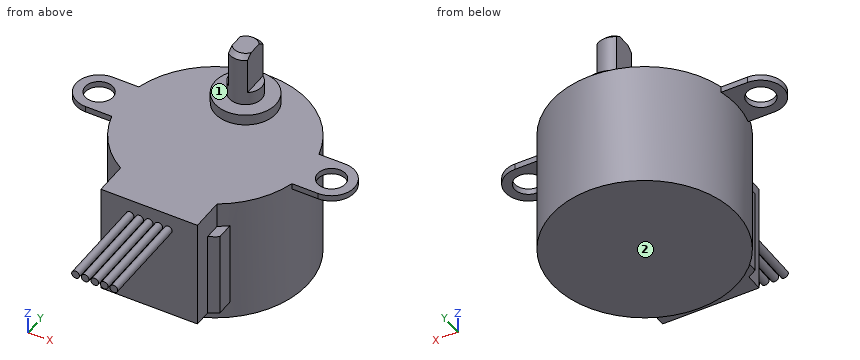
```python
from build123d import *

# Parameters (mm, degrees)
SKETCH1_R           = 14
BOSS_EXTRUDE1_DEPTH = 19.2
BOSS_EXTRUDE2_DEPTH = 16.64
BOSS_EXTRUDE3_DEPTH = 12.87
SKETCH4_R           = 0.585
BOSS_EXTRUDE4_DEPTH = 14
SKETCH5_R           = 4.6
BOSS_EXTRUDE5_DEPTH = 1.63
SKETCH6_R           = 2.445
BOSS_EXTRUDE6_DEPTH = 8.1
CUT_EXTRUDE1_DEPTH  = 6.08
CHAMFER1_SIZE       = 0.68
SKETCH8_R           = 2.1
BOSS_EXTRUDE7_DEPTH = 0.9


with BuildPart() as part:
    # Sketch1 → Boss-Extrude1 (new body)
    with BuildSketch(Plane.XY):
        Circle(SKETCH1_R)
    extrude(amount=-BOSS_EXTRUDE1_DEPTH)

    # Sketch2 → Boss-Extrude2 (add)
    with BuildSketch(Plane.XY):
        with BuildLine():
            Line((-7.265, -11.967446469), (-7.265, -17))
            Line((-7.265, -17), (7.265, -17))
            Line((7.265, -17), (7.265, -11.967446469))
            ThreePointArc((7.265, -11.967446469), (0, -14), (-7.265, -11.967446469))
        make_face()
    extrude(amount=-BOSS_EXTRUDE2_DEPTH)

    # Sketch3 → Boss-Extrude3 (add)
    with BuildSketch(Plane(origin=(0, 0, -16.64), x_dir=(-1, 0, 0), z_dir=(0, 0, -1))):
        with BuildLine():
            Line((7.265, -14.390072098), (7.265, -11.967446469))
            ThreePointArc((7.265, -11.967446469), (7.969331726, -11.510419273), (8.645, -11.011992327))
            Line((8.645, -11.011992327), (8.645, -13.605821364))
            ThreePointArc((8.645, -13.605821364), (7.964658643, -14.014942479), (7.265, -14.390072098))
        make_face()
        with BuildLine():
            Line((-7.265, -11.967446469), (-7.265, -14.390072098))
            ThreePointArc((-7.265, -14.390072098), (-7.964658643, -14.014942479), (-8.645, -13.605821364))
            Line((-8.645, -13.605821364), (-8.645, -11.011992327))
            ThreePointArc((-8.645, -11.011992327), (-7.969331726, -11.510419273), (-7.265, -11.967446469))
        make_face()
    extrude(amount=-BOSS_EXTRUDE3_DEPTH)

    # Sketch4 → Boss-Extrude4 (add)
    with BuildSketch(Plane.XZ.offset(17)):
        with Locations((-2.88, -2.555)):
            Circle(SKETCH4_R)
        with Locations((-1.44, -2.555)):
            Circle(SKETCH4_R)
        with Locations((0, -2.555)):
            Circle(SKETCH4_R)
        with Locations((1.44, -2.555)):
            Circle(SKETCH4_R)
        with Locations((2.88, -2.555)):
            Circle(SKETCH4_R)
    extrude(amount=BOSS_EXTRUDE4_DEPTH)

    # Sketch5 → Boss-Extrude5 (add)
    with BuildSketch(Plane.XY):
        with Locations((0, 7.77)):
            Circle(SKETCH5_R)
    extrude(amount=BOSS_EXTRUDE5_DEPTH)

    # Sketch6 → Boss-Extrude6 (add)
    with BuildSketch(Plane.XY.offset(1.63)):
        with Locations((0, 7.77)):
            Circle(SKETCH6_R)
    extrude(amount=BOSS_EXTRUDE6_DEPTH)

    # Sketch7 → Cut-Extrude1 (cut)
    with BuildSketch(Plane.XY.offset(9.73)):
        with BuildLine():
            Line((1.44, 9.745961791), (1.44, 5.794038209))
            ThreePointArc((1.44, 5.794038209), (2.445, 7.77), (1.44, 9.745961791))
        make_face()
        with BuildLine():
            Line((-1.44, 9.745961791), (-1.44, 5.794038209))
            ThreePointArc((-1.44, 5.794038209), (-2.445, 7.77), (-1.44, 9.745961791))
        make_face()
    extrude(amount=-CUT_EXTRUDE1_DEPTH, mode=Mode.SUBTRACT)

    # Chamfer1
    chamfer1_edges = [part.edges().sort_by_distance(p)[0] for p in [
        (0, 10.215, 9.73),
        (0, 5.325, 9.73),
    ]]
    chamfer(chamfer1_edges, length=CHAMFER1_SIZE)

    # Sketch8 → Boss-Extrude7 (add)
    with BuildSketch(Plane.XY):
        with BuildLine():
            Line((-13.561872105, 3.475), (-17.5, 3.475))
            ThreePointArc((-17.5, 3.475), (-20.975, 0), (-17.5, -3.475))
            Line((-17.5, -3.475), (-13.561872105, -3.475))
            ThreePointArc((-13.561872105, -3.475), (-14, 0), (-13.561872105, 3.475))
        make_face()
        with Locations((-17.5, 0)):
            Circle(SKETCH8_R, mode=Mode.SUBTRACT)
        with BuildLine():
            Line((17.5, -3.475), (13.561872105, -3.475))
            ThreePointArc((13.561872105, -3.475), (14, 0), (13.561872105, 3.475))
            Line((13.561872105, 3.475), (17.5, 3.475))
            ThreePointArc((17.5, 3.475), (20.975, 0), (17.5, -3.475))
        make_face()
        with Locations((17.5, 0)):
            Circle(SKETCH8_R, mode=Mode.SUBTRACT)
    extrude(amount=-BOSS_EXTRUDE7_DEPTH)


solid = part.part
```
Work out the finished part from the listing and answer in its coordinate system (mm). Face numbers are marked on the shaded views. A direction names the side the tool comes from. Give positions to 0.01 mm unless a question says otherwise; leave off trailing zeros. Loops run counter-clockwise (first coordinate to the right, second up) from the corner with the lowest first, then second, coordinate; pieces in that order, holes last. Notation, with made-up numbers: M 89.25,1 L 102.25,1 A25 cw 102.25,25 Z; hole C -12,-31 d9. An arc over 180 degrees is marked long. One line per item, written item: value. Start each with the question number.
1. Each of these flat-tipped pins is pushed along its axis until it touches: P1, Ø5, axis at y = 6, z = -6.5, coming from the -X side; P2, Ø1, axis at x = 16, z = -0.5, coming from the +Y side (3 decimals); P3, Ø2.5, axis at y = -15.5, z = -7.5, coming from the +X side. Where does it stop, or does it pass through?
2. Find the intervals of material crossed by probe 1 along Z at (x, y) = (-8, -2); probe 2 along Y at (x, z) = (-17.5, -0.35) (3 decimals); probe 3 along X at (y, z) = (-14.5, -12.5) (3 decimals), in increasing order.
3. Find section D-D (z = 5.25). Give the vertices of the cut face in (x, y) (3 decimals).
4. Find section A-A (x = 0). Give the vertices of the cut face in (y, z) (3 decimals), and give its area (3 significant figures).
5. Find section C-C (y = -21.5). Give the vertices of the cut face in (x, z) (3 decimals), and give its area (3 significant figures).
6. Find section B-B (x = 16.5). Give the vertices of the cut face in (y, z) (3 decimals), and give its area (3 significant figures).
7. Which of the six approach directions +Z, -Z, +X, -X, +Y, -Y give full straight-line access (tool end or side, diameter ignored) to the marked faces 1 and 2?
Reported:
1. P1: stops at x = -13.56
1. P2: stops at y = 3.475
1. P3: stops at x = 7.54
2. probe 1: z = -19.2 to 0
2. probe 2: y = -3.475 to -2.1, 2.1 to 3.475
2. probe 3: x = -7.265 to 7.265
3. outline: M -1.44,5.794 A2.445 ccw 1.44,5.794 L 1.44,9.746 A2.445 ccw -1.44,9.746 Z
4. outline: M -31,-3.14 L -17,-3.14 L -17,-16.64 L -14,-16.64 L -14,-19.2 L 14,-19.2 L 14,0 L 12.37,0 L 12.37,1.63 L 10.215,1.63 L 10.215,9.05 L 9.535,9.73 L 6.005,9.73 L 5.325,9.05 L 5.325,1.63 L 3.17,1.63 L 3.17,0 L -17,0 L -17,-1.97 L -31,-1.97 Z
4. area: 658 mm²
5. outline: C -2.88,-2.555 d1.17; C -1.44,-2.555 d1.17; C 0,-2.555 d1.17; C 1.44,-2.555 d1.17; C 2.88,-2.555 d1.17
5. area: 5.38 mm²
6. outline: M -3.475,-0.9 L -1.847,-0.9 L -1.847,0 L -3.475,0 Z; M 1.847,-0.9 L 3.475,-0.9 L 3.475,0 L 1.847,0 Z
6. area: 2.93 mm²
7. face 1: +Z
7. face 2: -Z, +X, -X, +Y, -Y
